Design review of the part built by this model. Coordinates are the model's own, in mm. Round coordinates to 2 decimals unless told otherwise and drop trailing zeros. Order: outer loops, then holes, each group sorted by start corner. A loop starts at its lowest first (then second) coordinate and runs counter-clockwise, first axis right, second up. Notation, with made-up numbers: M 21,-5 L 80,-5 A17 ccw 80,15 Z; hole C -21.75,42.25 d1. An arc over 180 degrees is marked long. Use a Markdown table: item, result. Add a question column.
(1) Take a section at C-C (z = 1.1). Write out the cut boundary in (x, y), then the cut area to 3 significant figures.
(2) To check wall thickness, follow probe 1 along Y at (x, z) = (-13, 1.8); probe 2 along X at (y, z) = (-34, 1); probe 3 along X at (y, z) = (-97.5, 2.55). State the ranges of each line that lie inside material, in increasing order. Write a range as from..to.
(3) Take a section at A-A (y = -40.5). Write out the cut boundary in (x, z), then the cut area to 3 significant figures.
(4) For pin 1 (4 mm diameter, centred on x = -47, y = 0, fed in from -Z), flat-tipped, find the tip position at first contact; note if it passes through.
(5) The part is to be moulded in two halves that separate along Y. For faces 1 (the face through (21.454, -98.918, 1.521)), 2 (the face through (0, -22, 3)), say which applies: released by +Y, released by -Y, zero draft, split by the parting line, or undercut.
(6) Take a section at B-B (x = -22). Write out the cut boundary in (y, z), then the cut area to 3 significant figures.
```python
from build123d import *

# Parameters (mm, degrees)
SKETCH1_W               = 141
SKETCH1_H               = 175
BOSS_EXTRUDE1_DEPTH     = 3
CUT_EXTRUDE1_DEPTH      = 132.816914117
CUT_EXTRUDE1_DEPTH_BACK = 132.816914117
SKETCH4_W               = 25.4
SKETCH4_H               = 19.05
SKETCH5_R               = 10
CUT_EXTRUDE2_DEPTH      = 132.816914117


with BuildPart() as part:
    # Sketch1 → Boss-Extrude1 (new body)
    with BuildSketch(Plane.XY):
        with Locations((1.330188679, -22.985849057)):
            Rectangle(SKETCH1_W, SKETCH1_H)
    extrude(amount=BOSS_EXTRUDE1_DEPTH)

    # Sketch4 → Cut-Extrude1 (cut, two sides: drawn at the far end of the back side and taken through both)
    with BuildSketch(Plane.XY.offset(3).offset(-CUT_EXTRUDE1_DEPTH_BACK)):
        with Locations((25.270813238, -37.985849057)):
            Rectangle(SKETCH4_W, SKETCH4_H)
        with Locations((25.270813238, -7.985849057)):
            Rectangle(SKETCH4_W, SKETCH4_H)
        with Locations((-24.729186762, -37.985849057)):
            Rectangle(SKETCH4_W, SKETCH4_H)
        with Locations((-24.729186762, -7.985849057)):
            Rectangle(SKETCH4_W, SKETCH4_H)
    extrude(amount=CUT_EXTRUDE1_DEPTH + CUT_EXTRUDE1_DEPTH_BACK, mode=Mode.SUBTRACT)

    # Sketch5 → Cut-Extrude2 (cut, through all)
    with BuildSketch(Plane.XY.offset(3)):
        with Locations((-24.169811321, -90.485849057)):
            Circle(SKETCH5_R)
        with Locations(Location((26.830188679, -90.485849057, 0), (0, 0, 180))):
            Circle(SKETCH5_R)
    extrude(amount=-CUT_EXTRUDE2_DEPTH, mode=Mode.SUBTRACT)


solid = part.part
```
Verdict:
| question | item | result |
|---|---|---|
| 1 | outline | M -69.17,-110.49 L 71.83,-110.49 L 71.83,64.51 L -69.17,64.51 Z; hole M -37.43,-47.51 L -12.03,-47.51 L -12.03,-28.46 L -37.43,-28.46 Z; hole M -37.43,-17.51 L -12.03,-17.51 L -12.03,1.54 L -37.43,1.54 Z; hole C -24.17,-90.49 d20; hole M 12.57,-47.51 L 37.97,-47.51 L 37.97,-28.46 L 12.57,-28.46 Z; hole M 12.57,-17.51 L 37.97,-17.51 L 37.97,1.54 L 12.57,1.54 Z; hole C 26.83,-90.49 d20 |
| 1 | area | 22,100 mm^2 |
| 2 | probe 1 | y = -110.49..-47.51, -28.46..-17.51, 1.54..64.51 |
| 2 | probe 2 | x = -69.17..-37.43, -12.03..12.57, 37.97..71.83 |
| 2 | probe 3 | x = -69.17..-31.3, -17.04..19.7, 33.96..71.83 |
| 3 | outline | M -69.17,0 L -37.43,0 L -37.43,3 L -69.17,3 Z; M -12.03,0 L 12.57,0 L 12.57,3 L -12.03,3 Z; M 37.97,0 L 71.83,0 L 71.83,3 L 37.97,3 Z |
| 3 | area | 271 mm^2 |
| 4 | pin 1 | stops at z = 0 |
| 5 | face 1 | undercut |
| 5 | face 2 | zero draft |
| 6 | outline | M -110.49,0 L -100.25,0 L -100.25,3 L -110.49,3 Z; M -80.72,0 L -47.51,0 L -47.51,3 L -80.72,3 Z; M -28.46,0 L -17.51,0 L -17.51,3 L -28.46,3 Z; M 1.54,0 L 64.51,0 L 64.51,3 L 1.54,3 Z |
| 6 | area | 352 mm^2 |
